from build123d import *

# Parameters (mm, degrees)
SKETCH1_R           = 2
SKETCH1_R_2         = 11
BOSS_EXTRUDE2_DEPTH = 3
FILLET1_R           = 50
SKETCH2_R           = 1.5
CUT_EXTRUDE1_DEPTH  = 10


with BuildPart() as part:
    # Sketch1 → Boss-Extrude2 (new body)
    with BuildSketch(Plane(origin=(0, 0, 0), x_dir=(1, 0, 0), z_dir=(0, 1, 0))):
        with BuildLine():
            Line((-43.210033531, -45.078612162), (230.077464987, -0.308197366))
            Line((230.077464987, -0.308197366), (291.16461822, -23.386663481))
            ThreePointArc((291.16461822, -23.386663481), (322.884028765, -10.065844598), (311.267854408, 22.316708024))
            Line((311.267854408, 22.316708024), (252.97547919, 51.748916229))
            Line((252.97547919, 51.748916229), (-51.951129031, 34.644890888))
            ThreePointArc((-51.951129031, 34.644890888), (-89.620314745, -9.826208081), (-43.210033531, -45.078612162))
        make_face()
        with Locations(Location((19.918584287, -11.5, 0), (0, 0, 270))):
            Circle(SKETCH1_R, mode=Mode.SUBTRACT)
        with Locations(Location((0, -23, 0), (0, 0, 270))):
            Circle(SKETCH1_R, mode=Mode.SUBTRACT)
        with Locations(Location((-19.918584287, -11.5, 0), (0, 0, 270))):
            Circle(SKETCH1_R, mode=Mode.SUBTRACT)
        with Locations(Location((-19.918584287, 11.5, 0), (0, 0, 270))):
            Circle(SKETCH1_R, mode=Mode.SUBTRACT)
        with Locations(Location((0, 23, 0), (0, 0, 270))):
            Circle(SKETCH1_R, mode=Mode.SUBTRACT)
        with Locations(Location((19.918584287, 11.5, 0), (0, 0, 270))):
            Circle(SKETCH1_R, mode=Mode.SUBTRACT)
        with Locations(Location((300, 0, 0), (0, 0, 270))):
            Circle(SKETCH1_R_2, mode=Mode.SUBTRACT)
    extrude(amount=BOSS_EXTRUDE2_DEPTH)

    # Fillet1
    fillet1_edges = [part.edges().sort_by_distance(p)[0] for p in [
        (252.97547919, 1.5, -51.748916229),
        (230.077464987, 1.5, 0.308197366),
    ]]
    fillet(fillet1_edges, radius=FILLET1_R)

    # Sketch2 → Cut-Extrude1 (cut)
    with BuildSketch(Plane(origin=(0, 3, 0), x_dir=(1, 0, 0), z_dir=(0, 1, 0))):
        with Locations(Location((-51.727112095, 30.651168763, 0), (0, 0, 270))):
            Circle(SKETCH2_R)
        with Locations(Location((-43.856700198, -41.13123047, 0), (0, 0, 270))):
            Circle(SKETCH2_R)
        with Locations(Location((-80.543038085, -24.356685052, 0), (0, 0, 270))):
            Circle(SKETCH2_R)
        with Locations(Location((-82.014474694, 11.465683169, 0), (0, 0, 270))):
            Circle(SKETCH2_R)
        with Locations(Location((-1.805585532, 33.451380461, 0), (0, 0, 270))):
            Circle(SKETCH2_R)
        with Locations(Location((48.115941032, 36.251592159, 0), (0, 0, 270))):
            Circle(SKETCH2_R)
        with Locations(Location((98.037467596, 39.051803857, 0), (0, 0, 270))):
            Circle(SKETCH2_R)
        with Locations(Location((147.958994159, 41.852015556, 0), (0, 0, 270))):
            Circle(SKETCH2_R)
        with Locations(Location((197.880520723, 44.652227254, 0), (0, 0, 270))):
            Circle(SKETCH2_R)
        with Locations(Location((247.802047287, 47.452438952, 0), (0, 0, 270))):
            Circle(SKETCH2_R)
        with Locations(Location((0.551343837, -33.85623047, 0), (0, 0, 270))):
            Circle(SKETCH2_R)
        with Locations(Location((44.959387872, -26.58123047, 0), (0, 0, 270))):
            Circle(SKETCH2_R)
        with Locations(Location((89.367431907, -19.30623047, 0), (0, 0, 270))):
            Circle(SKETCH2_R)
        with Locations(Location((133.775475942, -12.03123047, 0), (0, 0, 270))):
            Circle(SKETCH2_R)
        with Locations(Location((178.183519977, -4.75623047, 0), (0, 0, 270))):
            Circle(SKETCH2_R)
        with Locations(Location((222.591564011, 2.51876953, 0), (0, 0, 270))):
            Circle(SKETCH2_R)
    extrude(amount=-CUT_EXTRUDE1_DEPTH, mode=Mode.SUBTRACT)


solid = part.part
Work out the finished part from the listing and answer in its coordinate system (mm). A direction names the side the tool comes from. Coordinates: 2 decimals unless noted, no trailing zeros. Loops run counter-clockwise (first coordinate to the right, second up) from the corner with the lowest first, then second, coordinate; pieces in that order, holes last. Notation, with made-up numbers: M 34.5,48 L 90.5,48 A22 ccw 90.5,57 Z; hole C -32,50.5 d7. An arc over 180 degrees is marked long. Answer in a Markdown table with one row per item. Add a question column.
1. Flat-ended cylindrical pins translate along their axes: P1, Ø1.5, axis at x = 37.5, y = 2.5, coming from the -Z side; P2, Ø3.5, axis at x = 98.04, z = -39.05, coming from the +Y side. Find the tip coordinate at first contact, or state that the pin passes through.
2. Find section A-A, the plane y = 2.3. State how many separate pieces and enclosed holes the cut face has, then the cut area to 3 significant figures.
3. Find section B-B, the plane x = 13. Write down the section's boundary in (y, z), then the cut area to 3 significant figures.
4. Consider L1, parallel to Z at x = 248.5, y = 1.8; L2, parallel to Z at x = 291.5, y = 1; L3, parallel to Z at x = -48, y = 0.5. Determine where each line is inside the solid, lowest interval first.
5. Find section C-C, the plane x = 280.5. Write down the section's boundary in (y, z).
6. A tool of negligible diameter and unlimited length cuts with its end or side. For faces 4 (the flat face through (266.548, 1.479, 14.086)), 5 (the flat face through (115, 3, -3)), from which of +Z, -Z, +X, -X, +Y, -Y can it reach the whole face along a straight path? Write none if from no direction.
7. The mould has two halves that part along Z. Classify faces 1 (the cylindrical face through (310.906, 1.479, -1.432)), 2 (the flat face through (85.003, 1.479, 24.075)), 3 (the cylindrical face through (322.665, 1.479, 10.55)): pulls with the +Z half, pulls with the -Z half, needs draft (parallel to the pull), parting line crosses it, or undercut.
Reported:
| question | item | result |
|---|---|---|
| 1 | P1 | stops at z = -39.7 |
| 1 | P2 | stops at y = 3 |
| 2 | separate pieces | 1 |
| 2 | enclosed holes | 23 |
| 2 | area | 25,400 mm^2 |
| 3 | outline | M 0,-38.29 L 3,-38.29 L 3,35.87 L 0,35.87 Z |
| 3 | area | 222 mm^2 |
| 4 | L1 | z = -50.7 to -48.78, -46.12 to 7.27 |
| 4 | L2 | z = -32.3 to -6.98, 6.98 to 23.51 |
| 4 | L3 | z = -34.87 to 45.57 |
| 5 | outline | M 0,-37.85 L 3,-37.85 L 3,19.36 L 0,19.36 Z |
| 6 | face 4 | +Z, +Y, -Y |
| 6 | face 5 | +Z, -Z, +X, -X, +Y |
| 7 | face 1 | undercut |
| 7 | face 2 | pulls with the +Z half |
| 7 | face 3 | parting line crosses it |
